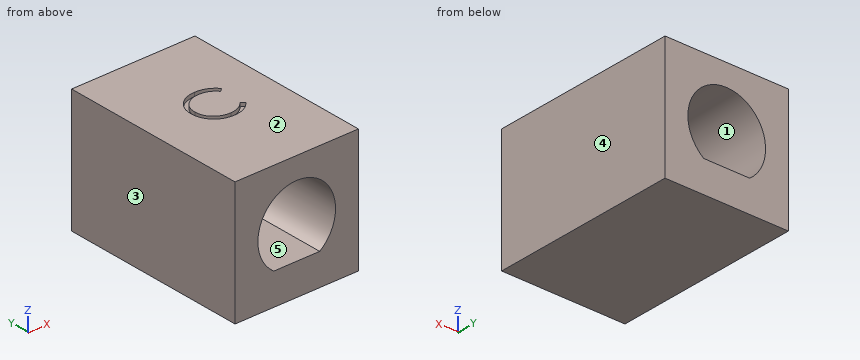
```python
from build123d import *

# Parameters (mm, degrees)
SKETCH1_W           = 9.84142284
SKETCH1_H           = 9.84142284
BOSS_EXTRUDE1_DEPTH = 15
CUT_EXTRUDE1_DEPTH  = 0.3


with BuildPart() as part:
    # Sketch1 → Boss-Extrude1 (new body)
    with BuildSketch(Plane(origin=(0, 0, 0), x_dir=(1, 0, 0), z_dir=(0, 1, 0))):
        Rectangle(SKETCH1_W, SKETCH1_H)
        with BuildLine():
            Line((-1.833030278, 2.409444822), (1.833030278, 2.409444822))
            ThreePointArc((1.833030278, 2.409444822), (0, -3.190555178), (-1.833030278, 2.409444822))
        make_face(mode=Mode.SUBTRACT)
    extrude(amount=BOSS_EXTRUDE1_DEPTH)

    # Sketch2 → Cut-Extrude1 (cut)
    with BuildSketch(Plane.XY.offset(4.92071142)):
        with BuildLine():
            Line((1.934406803, 9.11261109), (1.659567059, 8.902274552))
            add(Edge.make_bspline(
                [(1.659567059, 8.902274552), (1.639961171, 8.925640522), (1.601013724, 8.972057437), (1.538354521, 9.037236982), (1.473052878, 9.098302243), (1.405133757, 9.155544123), (1.333374638, 9.206960889), (1.259513839, 9.255231992), (1.182315794, 9.29849973), (1.075564059, 9.350962716), (0.935916211, 9.405708871), (0.760121372, 9.451612102), (0.576610273, 9.480833278), (0.451412674, 9.483998119), (0.387732123, 9.485607885)],
                knots=[0, 0, 0, 0, 9.1485e-05, 0.000181737, 0.000271024, 0.000359627, 0.000447979, 0.000535687, 0.000624217, 0.000713268, 0.000892422, 0.00107303, 0.001257466, 0.001448389, 0.001448389, 0.001448389, 0.001448389], degree=3))
            add(Edge.make_bspline(
                [(0.387732123, 9.485607885), (0.352648824, 9.485203923), (0.282807831, 9.484399747), (0.179159358, 9.473790622), (0.077446307, 9.458879412), (-0.02226516, 9.436754088), (-0.119848118, 9.408781469), (-0.21594052, 9.375356055), (-0.30915112, 9.334001215), (-0.400769358, 9.288292956), (-0.488548569, 9.236665511), (-0.571603617, 9.180352159), (-0.649631585, 9.119983062), (-0.722694197, 9.055331956), (-0.790866145, 8.986689996), (-0.853653456, 8.913325654), (-0.910838867, 8.83547348), (-0.963555892, 8.754160073), (-1.010768625, 8.669622281), (-1.050298504, 8.581547211), (-1.085303627, 8.491443108), (-1.113002869, 8.398291947), (-1.134927386, 8.302749181), (-1.150055049, 8.204558393), (-1.160543521, 8.103924714), (-1.161343697, 8.035715401), (-1.161747044, 8.001333045)],
                knots=[0, 0, 0, 0, 0.000105206, 0.000209435, 0.000312261, 0.00041348, 0.000515565, 0.000616682, 0.000718413, 0.000821258, 0.000923708, 0.001023662, 0.001122111, 0.001219464, 0.00131614, 0.001412112, 0.001508869, 0.001605718, 0.001702691, 0.001799013, 0.001895107, 0.001992482, 0.002090281, 0.00218895, 0.002290387, 0.00239349, 0.00239349, 0.00239349, 0.00239349], degree=3))
            add(Edge.make_bspline(
                [(-1.161747044, 8.001333045), (-1.160485225, 7.949601726), (-1.15800781, 7.848034141), (-1.135959476, 7.69926353), (-1.102454385, 7.556742856), (-1.052238808, 7.421363014), (-0.990319757, 7.291454656), (-0.912079146, 7.169215803), (-0.821462609, 7.052799238), (-0.717188189, 6.94495629), (-0.602782373, 6.846442565), (-0.480034462, 6.759691983), (-0.349250174, 6.687377101), (-0.211873544, 6.627201155), (-0.06684743, 6.580944427), (0.085567373, 6.548380303), (0.245039368, 6.527138123), (0.354008768, 6.525104435), (0.409466899, 6.524069424)],
                knots=[0, 0, 0, 0, 0.000155106, 0.000304531, 0.000450265, 0.000593548, 0.000736853, 0.000881182, 0.001028026, 0.001178769, 0.001330408, 0.001480379, 0.001628835, 0.001777978, 0.001929641, 0.002084627, 0.002245075, 0.00241136, 0.00241136, 0.00241136, 0.00241136], degree=3))
            add(Edge.make_bspline(
                [(0.409466899, 6.524069424), (0.470569588, 6.525758203), (0.590834297, 6.529082126), (0.767202323, 6.557241375), (0.936038089, 6.602899293), (1.097350675, 6.666797215), (1.250685321, 6.749862503), (1.396281982, 6.850560381), (1.534263552, 6.969848713), (1.617234834, 7.060931842), (1.659567059, 7.107402757)],
                knots=[0, 0, 0, 0, 0.00018322, 0.00036062, 0.000534275, 0.000707044, 0.000879893, 0.001056289, 0.001237208, 0.001425665, 0.001425665, 0.001425665, 0.001425665], degree=3))
            Line((1.659567059, 7.107402757), (1.934406803, 6.899169584))
            add(Edge.make_bspline(
                [(1.934406803, 6.899169584), (1.912288693, 6.870631132), (1.868158417, 6.813690926), (1.7967004, 6.733419216), (1.721423103, 6.65791518), (1.641767393, 6.587787559), (1.558649601, 6.521633094), (1.470577289, 6.461331262), (1.378708257, 6.406040378), (1.283353778, 6.355413454), (1.184615165, 6.310496207), (1.08261073, 6.272042439), (0.977780154, 6.238917549), (0.870118646, 6.211665612), (0.759402889, 6.190394529), (0.646032415, 6.176174854), (0.52976254, 6.166432939), (0.451321119, 6.165545024), (0.411570264, 6.165095065)],
                knots=[0, 0, 0, 0, 0.000108293, 0.000216068, 0.000322162, 0.000427957, 0.000534281, 0.00064066, 0.000747915, 0.000855806, 0.000964371, 0.001073102, 0.001182643, 0.001294024, 0.001406092, 0.001520624, 0.001636667, 0.001755891, 0.001755891, 0.001755891, 0.001755891], degree=3))
            add(Edge.make_bspline(
                [(0.411570264, 6.165095065), (0.373926597, 6.165357057), (0.299490907, 6.165875115), (0.189592155, 6.174267282), (0.082602575, 6.185717019), (-0.021172051, 6.20295715), (-0.122298026, 6.22330149), (-0.219858611, 6.250572747), (-0.314813821, 6.281121914), (-0.406782162, 6.3170269), (-0.495841862, 6.357543083), (-0.581705673, 6.403334642), (-0.664334105, 6.454016507), (-0.744539526, 6.508471517), (-0.82113711, 6.568448819), (-0.894790635, 6.633115453), (-0.965913112, 6.702253464), (-1.009915797, 6.752108317), (-1.032039512, 6.777174392)],
                knots=[0, 0, 0, 0, 0.0001129, 0.000223246, 0.000330481, 0.000435603, 0.000538732, 0.000639764, 0.000739316, 0.000837878, 0.000935767, 0.001032686, 0.001129604, 0.00122645, 0.001323362, 0.001421241, 0.001520399, 0.001620667, 0.001620667, 0.001620667, 0.001620667], degree=3))
            add(Edge.make_bspline(
                [(-1.032039512, 6.777174392), (-1.067475155, 6.82071558), (-1.137918632, 6.907272291), (-1.228044315, 7.047558272), (-1.305191871, 7.194026481), (-1.367567791, 7.34744641), (-1.416330525, 7.507473797), (-1.45011172, 7.674189311), (-1.472063324, 7.847437254), (-1.474573613, 7.965274042), (-1.475849608, 8.025171186)],
                knots=[0, 0, 0, 0, 0.000168306, 0.00033458, 0.000499224, 0.000664315, 0.00083066, 0.00100034, 0.001174094, 0.001353718, 0.001353718, 0.001353718, 0.001353718], degree=3))
            add(Edge.make_bspline(
                [(-1.475849608, 8.025171186), (-1.474294414, 8.08812664), (-1.471234668, 8.211987565), (-1.445238872, 8.393761518), (-1.403420076, 8.567912917), (-1.344023188, 8.734116661), (-1.268717836, 8.893246942), (-1.175691223, 9.044088146), (-1.06602408, 9.187604946), (-0.940576513, 9.321619697), (-0.803009177, 9.44415905), (-0.655690363, 9.551965254), (-0.498908416, 9.64168277), (-0.334390565, 9.716678932), (-0.160904883, 9.774323395), (0.021178486, 9.814676582), (0.211517401, 9.839793698), (0.341379826, 9.842968906), (0.407363533, 9.844582244)],
                knots=[0, 0, 0, 0, 0.000188789, 0.000371431, 0.000549644, 0.000725278, 0.00089996, 0.001076844, 0.001255917, 0.001440951, 0.001626689, 0.001807878, 0.001987546, 0.002167657, 0.002349462, 0.002534866, 0.002726448, 0.002924344, 0.002924344, 0.002924344, 0.002924344], degree=3))
            add(Edge.make_bspline(
                [(0.407363533, 9.844582244), (0.447578005, 9.844100106), (0.527178503, 9.843145762), (0.644931155, 9.83383962), (0.759573482, 9.818326014), (0.871184464, 9.797209944), (0.98030708, 9.771002622), (1.086107321, 9.736862324), (1.189206008, 9.697825793), (1.288952916, 9.652867327), (1.384869466, 9.602400585), (1.476925785, 9.546984962), (1.564390643, 9.486689156), (1.647879492, 9.422025981), (1.725995703, 9.351627422), (1.800957181, 9.277429826), (1.87021826, 9.197296001), (1.912971455, 9.140891068), (1.934406803, 9.11261109)],
                knots=[0, 0, 0, 0, 0.000120626, 0.000238766, 0.000354085, 0.000467531, 0.000579423, 0.000690512, 0.000800803, 0.000910007, 0.001018518, 0.001125773, 0.001232152, 0.001337058, 0.001442329, 0.001547432, 0.001653292, 0.001759736, 0.001759736, 0.001759736, 0.001759736], degree=3))
        make_face()
    extrude(amount=-CUT_EXTRUDE1_DEPTH, mode=Mode.SUBTRACT)


solid = part.part
```
Input: part model. Units: mm. Frame: model coordinates. Face numbers are marked on the shaded views. A direction names the side the tool comes from. Coordinates: 2 decimals unless noted, no trailing zeros. Write each loop counter-clockwise with the first axis right and the second up, starting at its lowest first coordinate (ties: lowest second). Pieces come first, ordered by that corner, then holes.
1) Mould query, pull axis X, two halves, no side actions, for the marked faces 1, 2 and 3. Classes: pulls with the +X half, pulls with the -X half, needs draft (parallel to the pull), parting line crosses it, or undercut.
2) Material intervals for line 1 along Z through (x, y) = (1.75, 11.5); line 2 along X through (y, z) = (8.75, 2); line 3 along Z through (x, y) = (-1, 13.25), sorted ascending.
3) Section C-C on x = 2.75. Output: boundary loops of the cut face in (y, z).
4) Section B-B on y = 2. Output: boundary loops of the cut face in (x, z), and give its area (3 significant figures).
5) Set-up query: the marked faces 4 and 5. Return all of +Z, -Z, +X, -X, +Y, -Y with unobstructed straight access to the full face (end or side cutting, diameter ignored); none if empty.
6) Section A-A on z = 1.5. Output: boundary loops of the cut face in (x, y).
Check result:
1. face 1: undercut
1. face 2: needs draft
1. face 3: pulls with the -X half
2. line 1: z = -4.92 to -2.41, 2.65 to 4.92
2. line 2: x = -4.92 to -2.44, 2.44 to 4.92
2. line 3: z = -4.92 to -2.41, 3.02 to 4.92
3. outline: (0, -4.92) - (15, -4.92) - (15, -1.34) - (0, -1.34) - close; (0, 1.52) - (15, 1.52) - (15, 4.92) - (0, 4.92) - close
4. outline: (-4.92, -4.92) - (4.92, -4.92) - (4.92, 4.92) - (-4.92, 4.92) - close; hole (-1.83, -2.41) - (1.83, -2.41) arc R3.1 ccw (long way) to start
4. area: 68.2 mm2
5. face 4: +Z, -Z, +X, +Y, -Y
5. face 5: +Y, -Y
6. outline: (-4.92, 0) - (-2.76, 0) - (-2.76, 15) - (-4.92, 15) - close; (2.76, 0) - (4.92, 0) - (4.92, 15) - (2.76, 15) - close
